Can you work these out from the model? Positions are in its coordinate system, mm. Face numbers are marked on the shaded views. A direction names the side the tool comes from. Give positions to 0.01 mm unless a question says otherwise; leave off trailing zeros. Order: outer loops, then holes, each group sorted by start corner. A loop starts at its lowest first (then second) coordinate and runs counter-clockwise, first axis right, second up. Notation, with made-up numbers: (43.25, 66) - (74.25, 66) arc R32 cw to (74.25, 96) - close; hole circle Ø4 at (-10, -21). An arc over 180 degrees is marked (long way). Use one line per item in the form item = value. Start each with the question number.
1) We'd pull the mould along Y, two halves only. Please class the marked faces 1, 2 and 3: released by +Y, released by -Y, zero draft, split by the parting line, or undercut.
2) Please list where these lines run through material, in increasing order: probe 1 along Z at (x, y) = (-18, 10.5); probe 2 along X at (y, z) = (25, 19.5); probe 3 along X at (y, z) = (11, 27.5).
3) Suppose I cut it at B-B, the plane z = 32.5. Write out the boundary of the cut face in (x, y).
4) Suppose I cut it at C-C, the plane y = 14. Write out the boundary of the cut face in (x, z), and give its area (3 significant figures).
5) Suppose I cut it at A-A, the plane x = 18. Write out the boundary of the cut face in (y, z), and give its area (3 significant figures).
6) Suppose I cut it at D-D, the plane z = 12. Write out the boundary of the cut face in (x, y), and give its area (3 significant figures).
7) For pin 1 (8 mm diameter, centred on x = -30, y = 23.5, fed in from +Z); pin 2 (12 mm diameter, centred on x = -7, y = 23.5, fed in from +Z); pin 3 (10 mm diameter, centred on x = -11.5, z = 22, fed in from -Y); pin 4 (6 mm diameter, centred on y = 29, z = 34.5, fed in from +X), each with a flat end and sliding along its axis, tell me the tip position at first contact or that it passes through.
8) Which directions (+Z, -Z, +X, -X, +Y, -Y) give clear straight access to the entire face, cutting with the end or side of a thin tool? Please do the marked faces 4, 5 and 6.
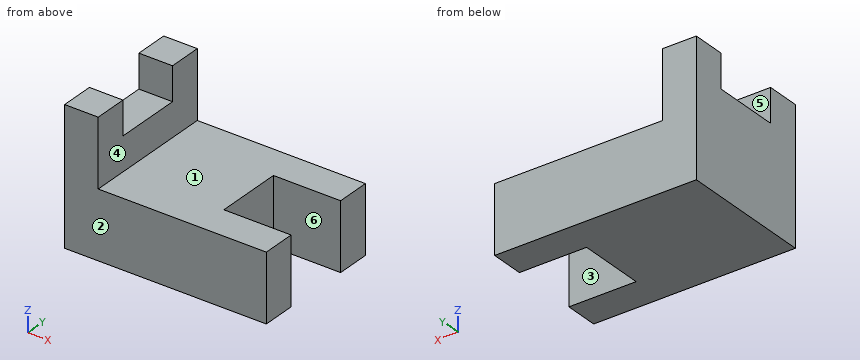
```python
from build123d import *

# Parameters (mm, degrees)
F0_W     = 60
F0_H     = 40
F1_DEPTH = 20
F3_W     = 10
F3_H     = 40
F4_DEPTH = 20
F5_W     = 20
F5_H     = 20
F6_DEPTH = 20.001
F7_W     = 10
F7_H     = 20
F8_DEPTH = 10


with BuildPart() as f1:
    # F0 (on Top) → F1 (new body)
    with BuildSketch(Plane.XY):
        with Locations((-7.431195, 20)):
            Rectangle(F0_W, F0_H)
    extrude(amount=F1_DEPTH)

    # F3 (on face) → F4 (join)
    with BuildSketch(Plane.XY.offset(20)):
        with Locations((-32.431195, 20)):
            Rectangle(F3_W, F3_H)
    extrude(amount=F4_DEPTH)

    # F5 (on face) → F6 (cut, through all)
    with BuildSketch(Plane.XY.offset(20)):
        with Locations((12.568805, 20)):
            Rectangle(F5_W, F5_H)
    extrude(amount=-F6_DEPTH, mode=Mode.SUBTRACT)

    # F7 (on face) → F8 (cut)
    with BuildSketch(Plane.XY.offset(40)):
        with Locations((-32.431195, 20)):
            Rectangle(F7_W, F7_H)
    extrude(amount=-F8_DEPTH, mode=Mode.SUBTRACT)


solid = f1.part
```
Result sheet:
q1.face_1 = zero draft
q1.face_2 = released by -Y
q1.face_3 = undercut
q2.probe_1 = 0 to 20
q2.probe_2 = -37.43 to 2.57
q2.probe_3 = -37.43 to -27.43
q3.outline = (-37.43, 0) - (-27.43, 0) - (-27.43, 10) - (-37.43, 10) - close; (-37.43, 30) - (-27.43, 30) - (-27.43, 40) - (-37.43, 40) - close
q4.outline = (-37.43, 0) - (2.57, 0) - (2.57, 20) - (-27.43, 20) - (-27.43, 30) - (-37.43, 30) - close
q4.area = 900 mm²
q5.outline = (0, 0) - (10, 0) - (10, 20) - (0, 20) - close; (30, 0) - (40, 0) - (40, 20) - (30, 20) - close
q5.area = 400 mm²
q6.outline = (-37.43, 0) - (22.57, 0) - (22.57, 10) - (2.57, 10) - (2.57, 30) - (22.57, 30) - (22.57, 40) - (-37.43, 40) - close
q6.area = 2,000 mm²
q7.pin_1 = 30
q7.pin_2 = 20
q7.pin_3 = 0
q7.pin_4 = -27.43
q8.face_4 = +Z, +X, +Y, -Y
q8.face_5 = +Z, +X, -X
q8.face_6 = +Z, -Z, +X
